Geometry: final body of the model. Coordinates: model frame, mm. A direction names the side the tool comes from. Coordinates: 2 decimals unless noted, no trailing zeros. Order: outer loops, then holes, each group sorted by start corner. A loop starts at its lowest first (then second) coordinate and runs counter-clockwise, first axis right, second up. Notation, with made-up numbers: M 45.25,9.5 L 56.25,9.5 A23 cw 56.25,39.5 Z; hole C -6.5,-31 d7. An arc over 180 degrees is marked long. Use CSV: the item, a comma, the result in double quotes. Start each with the question number.
Q1. Section query A-A, the plane y = 42. Output: boundary loops of the cut face in (x, z) (3 decimals), and give its area (3 significant figures).
Q2. Access query for faces 1 (the face through (1.61, 4.131, 35.365)), 2 (the face through (1.57, 234.94, 32.58)). Directions: +Z, -Z, +X, -X, +Y, -Y. A direction counts if a zero-diameter tool reaches every point of the face in a straight line with its end or side. Return the directions, or none.
Q3. Section query C-C, the plane x = 1.4. State how many separate pieces and enclosed holes the cut face has, and give its area (3 significant figures).
Q4. Section query B-B, the plane z = -8.5. Output: boundary loops of the cut face in (x, y) (3 decimals).
Q5. First-contact query: P1, Ø5, axis at y = 0, z = 0, coming from the +X side; P2, Ø1.6, axis at x = 1, y = 137.5, coming from the -Z side (3 decimals); P3, Ø1, axis at x = 2.5, y = 218.5, coming from the -Z side. Flat tips, straight axial feed; report the tip coordinate or a pass-through.
Q6. Mould query, pull axis Z, two halves, no side actions, for faces 3 (the face through (1.57, 175.91, 15.98)), 4 (the face through (1.565, 94.755, -34.277)), 5 (the face through (1.61, 33.86, 26.55)), 6 (the face through (0, 101, 24)). Classes: +Z half, -Z half, draft (parallel to the pull), parting line (faces both ways), or undercut.
Q7. Ray query, probe 1 along Y at (x, z) = (2, 44.45) (3 decimals); probe 2 along Z at (x, y) = (2.2, 119); probe 3 along Y at (x, z) = (1.35, 25.4). Return the intervals inside material, ascending.
Q8. Section query D-D, the plane z = 45. Output: boundary loops of the cut face in (x, y) (3 decimals).
from build123d import *

# Parameters (mm, degrees)
SKETCH1_R           = 3.175
BOSS_EXTRUDE1_DEPTH = 3.175
SKETCH2_W           = 19.05
SKETCH2_H           = 3.175
SKETCH2_W_2         = 12.7
CUT_EXTRUDE1_DEPTH  = 4.175
SKETCH3_R           = 23.810582085
SKETCH3_R_2         = 19.657709657
SKETCH3_R_3         = 16.108424526
SKETCH3_R_4         = 13.273253647
CUT_EXTRUDE2_DEPTH  = 4.175
SKETCH4_R           = 9.525
CUT_EXTRUDE3_DEPTH  = 4.175


with BuildPart() as part:
    # Sketch1 → Boss-Extrude1 (new body)
    with BuildSketch(Plane(origin=(0, 0, 0), x_dir=(0, 0, -1), z_dir=(1, 0, 0))):
        with BuildLine():
            Line((-69.85, 244.925264201), (5.752253277, 224.667701489))
            ThreePointArc((5.752253277, 224.667701489), (22.225, 203.2), (5.752253277, 181.732298511))
            Line((5.752253277, 181.732298511), (-38.324003746, 169.922101036))
            ThreePointArc((-38.324003746, 169.922101036), (-51.901174843, 160.850125345), (-57.15, 145.387585048))
            Line((-57.15, 145.387585048), (-57.15, -11.402464944))
            ThreePointArc((-57.15, -11.402464944), (-56.071518944, -18.725286548), (-52.927660139, -25.426255839))
            Line((-52.927660139, -25.426255839), (-35.988830069, -51.00598596))
            ThreePointArc((-35.988830069, -51.00598596), (-25.80648624, -56.687583685), (-15.281491626, -51.66910115))
            Line((-15.281491626, -51.66910115), (15.17776256, -11.512515957))
            ThreePointArc((15.17776256, -11.512515957), (17.524552025, -7.46944284), (18.816019124, -2.9765625))
            Line((18.816019124, -2.9765625), (50.176050998, 195.2625))
            ThreePointArc((50.176050998, 195.2625), (38.625542067, 236.195567884), (0, 254))
            Line((0, 254), (-69.85, 254))
            Line((-69.85, 254), (-69.85, 244.925264201))
        make_face()
        Circle(SKETCH1_R, mode=Mode.SUBTRACT)
        with Locations((-25.4, -43.994090512)):
            Circle(SKETCH1_R, mode=Mode.SUBTRACT)
        with BuildLine():
            Line((-24.4475, 158.75), (-24.4475, 57.15))
            ThreePointArc((-24.4475, 57.15), (-26.9875, 54.61), (-29.5275, 57.15))
            Line((-29.5275, 57.15), (-29.5275, 158.75))
            ThreePointArc((-29.5275, 158.75), (-26.9875, 161.29), (-24.4475, 158.75))
        make_face(mode=Mode.SUBTRACT)
    extrude(amount=BOSS_EXTRUDE1_DEPTH)

    # Sketch2 → Cut-Extrude1 (cut, through all)
    with BuildSketch(Plane.ZY):
        with Locations((44.45, 138.1125)):
            Rectangle(SKETCH2_W, SKETCH2_H)
        with Locations((34.925, 242.8875)):
            Rectangle(SKETCH2_W_2, SKETCH2_H)
    extrude(amount=-CUT_EXTRUDE1_DEPTH, mode=Mode.SUBTRACT)

    # Sketch3 → Cut-Extrude2 (cut, through all)
    with BuildSketch(Plane(origin=(3.175, 0, 0), x_dir=(0, 0, -1), z_dir=(1, 0, 0))):
        with Locations((8.888082085, 147.612778574)):
            Circle(SKETCH3_R)
        with Locations((4.735209657, 94.782459436)):
            Circle(SKETCH3_R_2)
        with Locations((1.185924526, 49.630611073)):
            Circle(SKETCH3_R_3)
        with Locations((-24.826746353, 20.698439358)):
            Circle(SKETCH3_R_4)
    extrude(amount=-CUT_EXTRUDE2_DEPTH, mode=Mode.SUBTRACT)

    # Sketch4 → Cut-Extrude3 (cut, through all)
    with BuildSketch(Plane(origin=(3.175, 0, 0), x_dir=(0, 0, -1), z_dir=(1, 0, 0))):
        with Locations((-44.45, 124.46)):
            Circle(SKETCH4_R)
        with Locations((-44.45, 1.27)):
            Circle(SKETCH4_R)
    extrude(amount=-CUT_EXTRUDE3_DEPTH, mode=Mode.SUBTRACT)


solid = part.part
Responses:
1,outline,"M 0,-25.931 L 3.175,-25.931 L 3.175,-15.372 L 0,-15.372 Z; M 0,13.001 L 3.175,13.001 L 3.175,57.15 L 0,57.15 Z"
1,area,"174 mm²"
2,face 1,"+X, -X"
2,face 2,"+Z, +X, -X"
3,separate pieces,"1"
3,enclosed holes,"11"
3,area,"16,700 mm²"
4,outline,"M 0,-20.316 L 3.175,-20.316 L 3.175,35.278 L 0,35.278 Z; M 0,63.983 L 3.175,63.983 L 3.175,75.489 L 0,75.489 Z; M 0,114.076 L 3.175,114.076 L 3.175,123.805 L 0,123.805 Z; M 0,171.42 L 3.175,171.42 L 3.175,182.665 L 0,182.665 Z; M 0,223.735 L 3.175,223.735 L 3.175,253.284 L 0,253.284 Z"
5,P1,"passes through"
5,P2,"stops at z = -41.165"
5,P3,"stops at z = -48.6"
6,face 3,"+Z half"
6,face 4,"-Z half"
6,face 5,"undercut"
6,face 6,"draft"
7,probe 1,"y = -38.229 to -8.255, 10.795 to 114.935, 133.985 to 136.525, 139.7 to 167.385, 238.119 to 254"
7,probe 2,"z = -38.11 to 24.45, 29.53 to 36.65, 52.25 to 57.15"
7,probe 3,"y = -56.69 to -47.17, -40.82 to 7.44, 33.96 to 55.17, 160.73 to 173.39, 233.01 to 254"
8,outline,"M 0,-37.398 L 3.175,-37.398 L 3.175,-8.239 L 0,-8.239 Z; M 0,10.779 L 3.175,10.779 L 3.175,114.951 L 0,114.951 Z; M 0,133.969 L 3.175,133.969 L 3.175,136.525 L 0,136.525 Z; M 0,139.7 L 3.175,139.7 L 3.175,167.058 L 0,167.058 Z; M 0,238.267 L 3.175,238.267 L 3.175,254 L 0,254 Z"
